```python
from build123d import *

# Parameters (mm, degrees)
CROQUIS1_W              = 203.31
CROQUIS1_H              = 67
SALIENTE_EXTRUIR1_DEPTH = 3
CORTAR_EXTRUIR1_REACH   = 5
CROQUIS2_W              = 10
CROQUIS2_H              = 20
CORTAR_EXTRUIR2_REACH   = 5
CROQUIS3_R              = 5


with BuildPart() as part:
    # Croquis1 → Saliente-Extruir1 (new body)
    with BuildSketch(Plane.XY):
        Rectangle(CROQUIS1_W, CROQUIS1_H)
    extrude(amount=-SALIENTE_EXTRUIR1_DEPTH)

    # Croquis2 → Cortar-Extruir1 (cut, up to next)
    with BuildSketch(Plane.XY, mode=Mode.PRIVATE) as cortar_extruir1_sk1:
        with Locations((-86.655, 13.5)):
            Rectangle(CROQUIS2_W, CROQUIS2_H)
    cortar_extruir1_tool1 = extrude(cortar_extruir1_sk1.sketch, amount=-CORTAR_EXTRUIR1_REACH, mode=Mode.PRIVATE) & part.part
    add(cortar_extruir1_tool1.solids().sort_by_distance((-86.655, 13.5, 0))[0], mode=Mode.SUBTRACT)

    # Croquis3 → Cortar-Extruir2 (cut, up to next)
    with BuildSketch(Plane.XY, mode=Mode.PRIVATE) as cortar_extruir2_sk1:
        with Locations((86.655, -18.5)):
            Circle(CROQUIS3_R)
    cortar_extruir2_tool1 = extrude(cortar_extruir2_sk1.sketch, amount=-CORTAR_EXTRUIR2_REACH, mode=Mode.PRIVATE) & part.part
    add(cortar_extruir2_tool1.solids().sort_by_distance((86.655, -18.5, 0))[0], mode=Mode.SUBTRACT)


solid = part.part
```
Work out the finished part from the listing and answer in its coordinate system (mm). Give positions to 0.01 mm unless a question says otherwise; leave off trailing zeros. Loops run counter-clockwise (first coordinate to the right, second up) from the corner with the lowest first, then second, coordinate; pieces in that order, holes last. Notation, with made-up numbers: M 55,5 L 98,5 A33 cw 98,41 Z; hole C -30.5,-16.5 d9. An arc over 180 degrees is marked long. One line per item, written item: value. Start each with the question number.
1. Determine the mould class of faces 1 (the face through (-1, 0, -3)), 2 (the face through (81.66, -18.28, -1.48)) for opening direction Y: released by +Y, released by -Y, zero draft, split by the parting line, or undercut.
2. Find section B-B (z = -0.85). Give the vertices of the cut face in (x, y) (3 decimals).
3. Find section A-A (y = -18.5). Give the vertices of the cut face in (x, z) (3 decimals), and give its area (3 significant figures).
4. Find the intervals of material crossed by probe 1 along X at (y, z) = (14.5, -2.8) (3 decimals), in increasing order.
Reported:
1. face 1: zero draft
1. face 2: undercut
2. outline: M -101.655,-33.5 L 101.655,-33.5 L 101.655,33.5 L -101.655,33.5 Z; hole M -91.655,3.5 L -81.655,3.5 L -81.655,23.5 L -91.655,23.5 Z; hole C 86.655,-18.5 d10
3. outline: M -101.655,-3 L 81.655,-3 L 81.655,0 L -101.655,0 Z; M 91.655,-3 L 101.655,-3 L 101.655,0 L 91.655,0 Z
3. area: 580 mm²
4. probe 1: x = -101.655 to -91.655, -81.655 to 101.655
